CAD build for the part. Positions are in the model's coordinates, mm. Round coordinates to 2 decimals unless told otherwise and drop trailing zeros. Order: outer loops, then holes, each group sorted by start corner. A loop starts at its lowest first (then second) coordinate and runs counter-clockwise, first axis right, second up. Notation, with made-up numbers: M 22.5,54 L 29.5,54 A16 cw 29.5,69 Z; hole C 7,82 d11. An arc over 180 degrees is marked long. Answer as a JSON object with one key per item and string values. Group by question number.
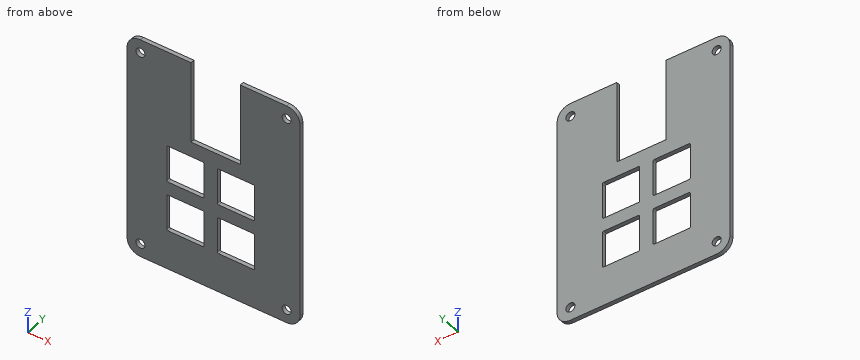
Autodesk Fusion 360 part; units mm, degrees
sketch "plate-2025-12-11T20_48_07.428Z" plane through (0, 0, 0) normal (0, 1, 0) x (1, 0, 0)
sketch "plate-2025-12-11T20_48_07.428Z (1)" plane through (0, 0, 0) normal (0, 1, 0) x (1, 0, 0)
  line L0 (3.025, -2.525) -> (16.025, -2.525)
  line L1 (3.025, -16.525) -> (16.025, -16.525)
  line L2 (2.525, -3.025) -> (2.525, -16.025)
  line L3 (16.525, -3.025) -> (16.525, -16.025)
  arc A0 (3.025, -2.525) -> (2.525, -3.025) centre (3.025, -3.025) ccw
  arc A1 (16.525, -3.025) -> (16.025, -2.525) centre (16.025, -3.025) ccw
  arc A2 (2.525, -16.025) -> (3.025, -16.525) centre (3.025, -16.025) ccw
  arc A3 (16.025, -16.525) -> (16.525, -16.025) centre (16.025, -16.025) ccw
  line L4 (22.075, -2.525) -> (35.075, -2.525)
  line L5 (22.075, -16.525) -> (35.075, -16.525)
  line L6 (21.575, -3.025) -> (21.575, -16.025)
  line L7 (35.575, -3.025) -> (35.575, -16.025)
  arc A4 (22.075, -2.525) -> (21.575, -3.025) centre (22.075, -3.025) ccw
  arc A5 (35.575, -3.025) -> (35.075, -2.525) centre (35.075, -3.025) ccw
  arc A6 (21.575, -16.025) -> (22.075, -16.525) centre (22.075, -16.025) ccw
  arc A7 (35.075, -16.525) -> (35.575, -16.025) centre (35.075, -16.025) ccw
  line L8 (3.025, -21.575) -> (16.025, -21.575)
  line L9 (3.025, -35.575) -> (16.025, -35.575)
  line L10 (2.525, -22.075) -> (2.525, -35.075)
  line L11 (16.525, -22.075) -> (16.525, -35.075)
  arc A8 (3.025, -21.575) -> (2.525, -22.075) centre (3.025, -22.075) ccw
  arc A9 (16.525, -22.075) -> (16.025, -21.575) centre (16.025, -22.075) ccw
  arc A10 (2.525, -35.075) -> (3.025, -35.575) centre (3.025, -35.075) ccw
  arc A11 (16.025, -35.575) -> (16.525, -35.075) centre (16.025, -35.075) ccw
  line L12 (22.075, -21.575) -> (35.075, -21.575)
  line L13 (22.075, -35.575) -> (35.075, -35.575)
  line L14 (21.575, -22.075) -> (21.575, -35.075)
  line L15 (35.575, -22.075) -> (35.575, -35.075)
  arc A12 (22.075, -21.575) -> (21.575, -22.075) centre (22.075, -22.075) ccw
  arc A13 (35.575, -22.075) -> (35.075, -21.575) centre (35.075, -22.075) ccw
  arc A14 (21.575, -35.075) -> (22.075, -35.575) centre (22.075, -35.075) ccw
  arc A15 (35.075, -35.575) -> (35.575, -35.075) centre (35.075, -35.075) ccw
sketch "Sketch5" plane through (0, 0, 0) normal (0, 1, 0) x (1, 0, 0)
  line L0 (-12.375, -72.225) -> (52.625, -72.225)
  line L1 (52.625, -72.225) -> (52.625, 12.375)
  line L2 (52.625, 12.375) -> (-12.375, 12.375)
  line L3 (-12.375, 12.375) -> (-12.375, -72.225)
  line L4 (3.025, -2.525) -> (16.025, -2.525)
  line L5 (2.525, -3.025) -> (2.525, -16.025)
  line L6 (11.68, -72.225) -> (30.18, -72.225)
  line L7 (30.18, -72.225) -> (30.18, -41.225)
  line L8 (30.18, -41.225) -> (11.68, -41.225)
  line L9 (11.68, -41.225) -> (11.68, -72.225)
  circle A0 centre (-7.375, -67.225) radius 1.7
  circle A1 centre (47.625, -67.225) radius 1.7
  circle A2 centre (47.625, 7.375) radius 1.7
  circle A3 centre (-7.375, 7.375) radius 1.7
  dimension "d1" = 84.6
  dimension "d2" = 65
  dimension "d3" = 14.9
  dimension "d4" = 14.9
  dimension "d5" = 31
  dimension "d6" = 18.5
  dimension "d7" = 24.055
  dimension "d8" = 3.4
  dimension "d9" = 5
  dimension "d10" = 3.4
  dimension "d11" = 5
  dimension "d12" = 3.4
  dimension "d13" = 5
  dimension "d14" = 3.4
  dimension "d15" = 5
  dimension "d16" = 5
  dimension "d17" = 5
  dimension "d18" = 5
  dimension "d19" = 5
extrude "Extrude1" add sketch "Sketch5" along normal blind 1.5 contours L0 L1 L2 L3 L7 L8 L9
extrude "Extrude2" cut sketch "plate-2025-12-11T20_48_07.428Z (1)" along normal through all
fillet "Fillet1" radius 5 4 edges at (-12.375, 0.75, 72.225) (52.625, 0.75, 72.225) (52.625, 0.75, -12.375) (-12.375, 0.75, -12.375)
Item 1: Cut at D-D, the plane y = 1.15. Give the number of separate pieces and of enclosed holes in the cut face, and give its area (3 significant figures).
Item 2: Cut at A-A, the plane z = 61.5. Give the cut face in (x, y) (3 decimals), and give its area (4 significant figures).
Item 3: Cut at B-B, the plane x = 6.5. Give the cut face in (y, z) (3 decimals), and give its area (3 significant figures).
Item 4: Drill centre lines: line 1 (Z direction, x = 33, y = 0.4) (3 decimals); line 2 (X direction, y = 1.1, z = 11) (3 decimals); line 3 (Z direction, x = 12.5, y = 0.1) (3 decimals). Where is each one in solid material? Low to high. Write a range as [from, to].
Item 5: Cut at C-C, the plane z = 32.5. Give the cut face in (x, y) (3 decimals).
Response values:
{
 "1": {"separate pieces": "1", "enclosed holes": "8", "area": "4,080 mm^2"},
 "2": {"outline": "M -12.375,0 L 11.68,0 L 11.68,1.5 L -12.375,1.5 Z; M 30.18,0 L 52.625,0 L 52.625,1.5 L 30.18,1.5 Z", "area": "69.75 mm^2"},
 "3": {"outline": "M 0,-12.375 L 1.5,-12.375 L 1.5,2.525 L 0,2.525 Z; M 0,16.525 L 1.5,16.525 L 1.5,21.575 L 0,21.575 Z; M 0,35.575 L 1.5,35.575 L 1.5,72.225 L 0,72.225 Z", "area": "84.9 mm^2"},
 "4": {"line 1": "[-12.375, 2.525], [16.525, 21.575], [35.575, 72.225]", "line 2": "[-12.375, 2.525], [16.525, 21.575], [35.575, 52.625]", "line 3": "[-12.375, 2.525], [16.525, 21.575], [35.575, 41.225]"},
 "5": {"outline": "M -12.375,0 L 2.525,0 L 2.525,1.5 L -12.375,1.5 Z; M 16.525,0 L 21.575,0 L 21.575,1.5 L 16.525,1.5 Z; M 35.575,0 L 52.625,0 L 52.625,1.5 L 35.575,1.5 Z"}
}
